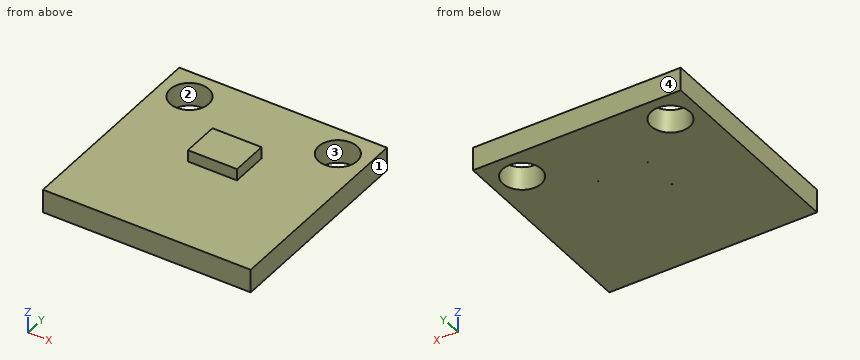
from build123d import *

# Parameters (mm, degrees)
MODEL_R             = 1.651
MODEL_W             = 4.1999916
MODEL_H             = 3.1999936
BOSS_EXTRUDE1_DEPTH = 2
MODEL_3_W           = 4.1999916
MODEL_3_H           = 3.1999936
BOSS_EXTRUDE2_DEPTH = 3


with BuildPart() as part:
    # Model → Boss-Extrude1 (new body)
    # profile 1 of 2: a face of its own
    with BuildSketch(Plane.XY):
        Polygon((0, 0.0508), (0, 0), (0.0508, 0), (17.7292, 0), (17.78, 0), (17.78, 0.0508), (17.78, 17.7292), (17.78, 17.78), (17.7292, 17.78), (0.0508, 17.78), (0, 17.78), (0, 17.7292), align=None)
        with Locations((2.54, 15.24)):
            Circle(MODEL_R, mode=Mode.SUBTRACT)
        with BuildLine():
            Line((10.9582458, 8.5600032), (6.8217542, 8.5600032))
            ThreePointArc((6.8217542, 8.5600032), (6.81245484, 8.53755256), (6.7900042, 8.5282532))
            ThreePointArc((6.7900042, 8.5282532), (6.76755356, 8.53755256), (6.7582542, 8.5600032))
            ThreePointArc((6.7582542, 8.5600032), (6.76755356, 8.58245384), (6.7900042, 8.5917532))
            Line((6.7900042, 8.5917532), (6.7900042, 11.7282468))
            ThreePointArc((6.7900042, 11.7282468), (6.76755356, 11.73754616), (6.7582542, 11.7599968))
            ThreePointArc((6.7582542, 11.7599968), (6.76755356, 11.78244744), (6.7900042, 11.7917468))
            ThreePointArc((6.7900042, 11.7917468), (6.81245484, 11.78244744), (6.8217542, 11.7599968))
            Line((6.8217542, 11.7599968), (10.9582458, 11.7599968))
            ThreePointArc((10.9582458, 11.7599968), (10.96754516, 11.78244744), (10.9899958, 11.7917468))
            ThreePointArc((10.9899958, 11.7917468), (11.01244644, 11.78244744), (11.0217458, 11.7599968))
            ThreePointArc((11.0217458, 11.7599968), (11.01244644, 11.73754616), (10.9899958, 11.7282468))
            Line((10.9899958, 11.7282468), (10.9899958, 8.5917532))
            ThreePointArc((10.9899958, 8.5917532), (11.01244644, 8.58245384), (11.0217458, 8.5600032))
            ThreePointArc((11.0217458, 8.5600032), (11.01244644, 8.53755256), (10.9899958, 8.5282532))
            ThreePointArc((10.9899958, 8.5282532), (10.96754516, 8.53755256), (10.9582458, 8.5600032))
        make_face(mode=Mode.SUBTRACT)
        with Locations((15.24, 15.24)):
            Circle(MODEL_R, mode=Mode.SUBTRACT)
    # profile 2 of 2: a face of its own
    with BuildSketch(Plane.XY):
        with Locations((8.89, 10.16)):
            Rectangle(MODEL_W, MODEL_H)
    extrude(amount=BOSS_EXTRUDE1_DEPTH)

    # Model_3 → Boss-Extrude2 (add)
    with BuildSketch(Plane.XY):
        with Locations((8.89, 10.16)):
            Rectangle(MODEL_3_W, MODEL_3_H)
    extrude(amount=BOSS_EXTRUDE2_DEPTH)


solid = part.part
The model under review builds one solid part; all positions refer to its coordinate system, in mm. Face numbers are marked on the shaded views. Coordinates: 2 decimals unless noted, no trailing zeros. Loops run counter-clockwise (first coordinate to the right, second up) from the corner with the lowest first, then second, coordinate; pieces in that order, holes last. Notation, with made-up numbers: M -1.75,49 L 49.25,49 A31 ccw 49.25,80 Z; hole C 22,-24 d8. An arc over 180 degrees is marked long. Put each result on its own line as item: value. Start each with the question number.
Q1. Add section A-A (y = 15.24). Write out the cut boundary in (x, z), and give its area (3 significant figures).
Q2. Clearance check with flat-ended pins moving along their axes: pin 1 (1 mm diameter, centred on x = 4.5, y = 6.5, fed in from -Z); pin 2 (2 mm diameter, centred on x = 15.24, y = 15.24, fed in from -Z); pin 3 (1 mm diameter, centred on x = 7.5, y = 2, fed in from +Z). State where each tip first meets the part, or that it passes through.
Q3. Wall thickness on line 1 (X direction, y = 15.25, z = 0.5); line 2 (Y direction, x = 15.24, z = 0.8); line 3 (Y direction, x = 8, z = 2.05): over which ranges is each line inside the solid? List them lowest first.
Q4. The part is to be moulded in two halves that separate along X. For the marked faces 1, 2, 3 and 4, say which applies: +X half, -X half, draft (parallel to the pull), parting line (faces both ways), or undercut.
Q5. Add section B-B (x = 15.24). Write out the cut boundary in (y, z), and give its area (3 significant figures).
Q6. Add section D-D (z = 2.5). Write out the cut boundary in (x, y), and give its area (3 significant figures).
Q7. Add section C-C (y = 2.25). Write out the cut boundary in (x, z), and give its area (3 significant figures).
Answers:
1. outline: M 0,0 L 0.89,0 L 0.89,2 L 0,2 Z; M 4.19,0 L 13.59,0 L 13.59,2 L 4.19,2 Z; M 16.89,0 L 17.78,0 L 17.78,2 L 16.89,2 Z
1. area: 22.4 mm^2
2. pin 1: stops at z = 0
2. pin 2: passes through
2. pin 3: stops at z = 2
3. line 1: x = 0 to 0.89, 4.19 to 13.59, 16.89 to 17.78
3. line 2: y = 0 to 13.59, 16.89 to 17.78
3. line 3: y = 8.56 to 11.76
4. face 1: +X half
4. face 2: undercut
4. face 3: undercut
4. face 4: draft
5. outline: M 0,0 L 13.59,0 L 13.59,2 L 0,2 Z; M 16.89,0 L 17.78,0 L 17.78,2 L 16.89,2 Z
5. area: 29.0 mm^2
6. outline: M 6.79,8.56 L 10.99,8.56 L 10.99,11.76 L 6.79,11.76 Z
6. area: 13.4 mm^2
7. outline: M 0,0 L 17.78,0 L 17.78,2 L 0,2 Z
7. area: 35.6 mm^2
